from build123d import *

# Parameters (mm, degrees)
BOX081_W     = 9.5
BOX081_H     = 12.95
BOX081_DEPTH = 1.1
BOX080_W     = 9.5
BOX080_H     = 13
BOX080_DEPTH = 1.2


with BuildPart() as small_cu_gnd_electrode026:
    # Box081 → Box081 (new body)
    with BuildSketch(Plane.XY.offset(0.05)):
        with Locations((4.75, 6.475)):
            Rectangle(BOX081_W, BOX081_H)
    extrude(amount=BOX081_DEPTH)


with BuildPart() as large_cu_electrode_long_axis_v_y:
    # Box080 → Box080 (new body)
    with BuildSketch(Plane.XY):
        with Locations((4.75, 6.5)):
            Rectangle(BOX080_W, BOX080_H)
    extrude(amount=BOX080_DEPTH)

    # Cut026: cut Small Cu GND Electrode026
    add(small_cu_gnd_electrode026.part, mode=Mode.SUBTRACT)


with BuildPart() as large_cu_electrode_long_axis_v_y_1:
    # Cut026 placement: moved
    add(large_cu_electrode_long_axis_v_y.part.moved(Location((-4.76, 9.63, 21.1))))


solid = large_cu_electrode_long_axis_v_y_1.part
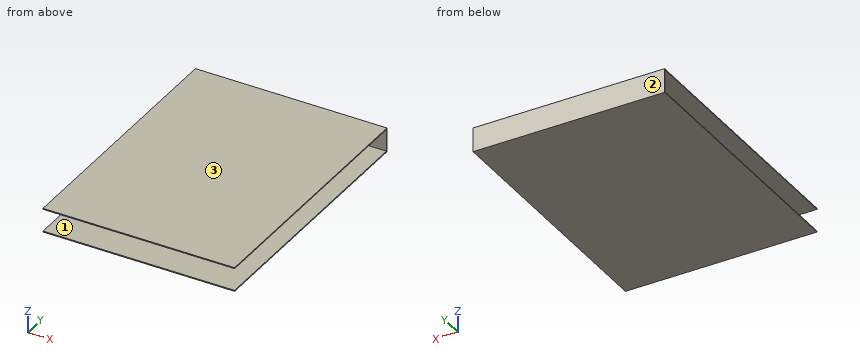
Part model, mm, in its own coordinate system. Face numbers are marked on the shaded views. Round coordinates to 2 decimals unless told otherwise and drop trailing zeros. Loops run counter-clockwise (first coordinate to the right, second up) from the corner with the lowest first, then second, coordinate; pieces in that order, holes last. Notation, with made-up numbers: (73.5, -26) - (112.5, -26) arc R18 cw to (112.5, 6) - close; hole circle Ø1 at (85, 4.5). An arc over 180 degrees is marked (long way). Answer as a JSON object with one key per item and string values.
Item 1: Band-saw the part on A-A on y = 19. List the corners of the cut face in (x, z).
Output:
{"outline": "(-4.76, 21.1) - (4.74, 21.1) - (4.74, 21.15) - (-4.76, 21.15) - close; (-4.76, 22.25) - (4.74, 22.25) - (4.74, 22.3) - (-4.76, 22.3) - close"}
Item 2: Band-saw the part on B-B on x = 0.5. List the corners of the cut face in (y, z), plus the area to 4 significant figures.
Output:
{"outline": "(9.63, 21.1) - (22.63, 21.1) - (22.63, 22.3) - (9.63, 22.3) - (9.63, 22.25) - (22.58, 22.25) - (22.58, 21.15) - (9.63, 21.15) - close", "area": "1.355 mm2"}
Item 3: Pin check, flat tip, straight feed: pin 1 (0.6 mm diameter, centred on x = -0.5, z = 21.5, fed in from -Y). Stop position of the tip, or through.
Output:
{"pin 1": "y = 22.58"}
Item 4: Band-saw the part on C-C on z = 21.8. List the corners of the cut face in (x, y).
Output:
{"outline": "(-4.76, 22.58) - (4.74, 22.58) - (4.74, 22.63) - (-4.76, 22.63) - close"}
Item 5: Pull direction Z, two halves, no side cores. Call the marked faces 1, 2 and 3: pulls with the +Z half, pulls with the -Z half, needs draft (parallel to the pull), parting line crosses it, or undercut.
Output:
{"face 1": "undercut", "face 2": "needs draft", "face 3": "pulls with the +Z half"}
